from build123d import *

# Parameters (mm, degrees)
F1_DEPTH       = 10
F3_D           = 5
F3_CBORE_D     = 9
F3_CBORE_DEPTH = 1.5
F4_T1_DEPTH    = 10
F4_T3_DEPTH    = 10
F4_T5_DEPTH    = 10
F4_T7_DEPTH    = 35
F4_T9_DEPTH    = 35
F4_T11_DEPTH   = 35
F4_T13_DEPTH   = 34.4948974279
F5_R           = 2


# Not quite as in the source:
# - a fillet or chamfer that OpenCascade refuses, or shapes differently, is made with other operations: its cross-section is extruded or revolved along the edge and cut away or added


with BuildPart() as f1:
    # F0 (on Top) → F1 (new body)
    with BuildSketch(Plane.XY):
        Polygon((-60, 0), (0, 0), (0, 7), (-54, 7), (-54, 22), (-20, 22), (-20, 11), (-16, 11), (-16, 28), (-60, 28), align=None)
    extrude(amount=F1_DEPTH)

    # F3 (through all)
    with Locations(Plane(origin=(0, 7, 0), x_dir=(-1, 0, 0), z_dir=(0, 1, 0))):
        with Locations((8, 5)):
            CounterBoreHole(F3_D / 2, F3_CBORE_D / 2, F3_CBORE_DEPTH)

    # F4: fillet of radius 5 on 7 edges, made by hand

    # F4_s2 → F4_t1 (join)
    with BuildSketch(Plane.XY):
        with BuildLine():
            ThreePointArc((-49, 7), (-52.5355339059, 8.4644660941), (-54, 12))
            Line((-54, 12), (-54, 7))
            Line((-54, 7), (-49, 7))
        make_face()
    extrude(amount=F4_T1_DEPTH)

    # F4_s4 → F4_t3 (join)
    with BuildSketch(Plane.XY):
        with BuildLine():
            ThreePointArc((-54, 17), (-52.5355339059, 20.5355339059), (-49, 22))
            Line((-49, 22), (-54, 22))
            Line((-54, 22), (-54, 17))
        make_face()
    extrude(amount=F4_T3_DEPTH)

    # F4_s6 → F4_t5 (join)
    with BuildSketch(Plane.XY):
        with BuildLine():
            ThreePointArc((-25, 22), (-21.4644660941, 20.5355339059), (-20, 17))
            Line((-20, 17), (-20, 22))
            Line((-20, 22), (-25, 22))
        make_face()
    extrude(amount=F4_T5_DEPTH)

    # F4_s8 → F4_t7 (cut)
    with BuildSketch(Plane.XY.offset(-12.5)):
        with BuildLine():
            ThreePointArc((-55, 0), (-58.5355339059, 1.4644660941), (-60, 5))
            Line((-60, 5), (-60, 0))
            Line((-60, 0), (-55, 0))
        make_face()
    extrude(amount=F4_T7_DEPTH, mode=Mode.SUBTRACT)

    # F4_s10 → F4_t9 (cut)
    with BuildSketch(Plane.XY.offset(-12.5)):
        with BuildLine():
            ThreePointArc((-60, 23), (-58.5355339059, 26.5355339059), (-55, 28))
            Line((-55, 28), (-60, 28))
            Line((-60, 28), (-60, 23))
        make_face()
    extrude(amount=F4_T9_DEPTH, mode=Mode.SUBTRACT)

    # F4_s12 → F4_t11 (cut)
    with BuildSketch(Plane.XY.offset(-12.5)):
        with BuildLine():
            ThreePointArc((-21, 28), (-17.4644660941, 26.5355339059), (-16, 23))
            Line((-16, 23), (-16, 28))
            Line((-16, 28), (-21, 28))
        make_face()
    extrude(amount=F4_T11_DEPTH, mode=Mode.SUBTRACT)

    # F4_s14 → F4_t13 (cut)
    with BuildSketch(Plane.XY.offset(-12.2474487139)):
        with BuildLine():
            ThreePointArc((-16, 15.8989794856), (-17.1270166538, 12.7367018254), (-20, 11))
            Line((-20, 11), (-16, 11))
            Line((-16, 11), (-16, 15.8989794856))
        make_face()
    extrude(amount=F4_T13_DEPTH, mode=Mode.SUBTRACT)

    # F5
    f5_edges = [f1.edges().sort_by_distance(p)[0] for p in [
        (-38, 28, 0),
        (-55, 28, 5),
        (-38, 28, 10),
        (-21, 28, 5),
        (-16, 19.44949, 0),
        (-16, 19.44949, 10),
        (-60, 14, 0),
        (-60, 14, 10),
        (-27.5, 0, 0),
        (-27.5, 0, 10),
        (-58.535534, 1.464466, 0),
        (-58.535534, 26.535534, 0),
        (-17.464466, 26.535534, 0),
        (-17.127017, 12.736702, 0),
        (-58.535534, 1.464466, 10),
        (-58.535534, 26.535534, 10),
        (-17.464466, 26.535534, 10),
        (-17.127017, 12.736702, 10),
    ]]
    fillet(f5_edges, radius=F5_R)


solid = f1.part
Could you check a few things on this model? Use its own coordinates, in mm. A direction names the side the tool comes from. Give positions to 0.01 mm unless a question says otherwise; leave off trailing zeros. Order: outer loops, then holes, each group sorted by start corner. A loop starts at its lowest first (then second) coordinate and runs counter-clockwise, first axis right, second up. Notation, with made-up numbers: (56.5, 60.25) - (88.5, 60.25) arc R16 cw to (88.5, 85.25) - close; hole circle Ø2 at (26.25, 35.5). An arc over 180 degrees is marked (long way). One line per question, with ' | ' between items. Start each with the question number.
Item 1: I want a section at A-A on z = 5. Write out the boundary of the cut face in (x, y), then the cut area to 3 significant figures.
Item 2: I want a section at B-B on x = -47. Write out the boundary of the cut face in (y, z), then the cut area to 3 significant figures.
Item 3: I want a section at D-D on x = -8. Write out the boundary of the cut face in (y, z), then the cut area to 3 significant figures.
Item 4: For faces 4 (the cylindrical face through (-16.6, 19.5, 0.57)), 5 (the cylindrical face through (-12.16, 6.26, 3.28)), 6 (the flat face through (-16, 19, 5)), 7 (the cylindrical face through (-17.1, 12.77, 4.96)), 8 (the flat face through (-20, 14, 5)), which set-ups out of +Z, -Z, +X, -X, +Y, -Y let a thin tool reach every point of the face, with its end or its side?
Item 5: I'm going to push flat-ended pins straight in: pin 1 Ø4 at (y, z) = (23.5, 6.5) entering from +X; pin 2 Ø4 at (x, z) = (-51, 5) entering from -Y; pin 3 Ø2.5 at (x, z) = (-10, 6.5) entering from +Y; pin 4 Ø5 at (x, z) = (-14.5, 6.5) entering from +Y. Where does each tip first touch, or does it pass through?
Item 6: I want a section at C-C on y = 20.75. Write out the boundary of the cut face in (x, z).
Item 7: I need wall thicknesses on probe 1 along Z at (x, y) = (-8, 2.85); probe 2 along Y at (x, z) = (-39.5, 2.5); probe 3 along Z at (x, y) = (-8, 6.2). Which ranges of each line are inside material? Lowest first, please. Write a range as [from, to].
Item 8: Thinking about a two-plate mould opening in Y: for faces 1 (the cylindrical face through (-9.84, 2.71, 6.69)), 2 (the cylindrical face through (-53, 20, 5)), 3 (the flat face through (-10, 5.5, 3)), which applies, pulls with the +Y half, pulls with the -Y half, needs draft (parallel to the pull), parting line crosses it, or undercut?
Verdict:
1) outline: (-60, 5) arc R5 ccw to (-55, 0) - (-10.5, 0) - (-10.5, 5.5) - (-12.5, 5.5) - (-12.5, 7) - (-49, 7) arc R5 cw to (-54, 12) - (-54, 17) arc R5 cw to (-49, 22) - (-25, 22) arc R5 cw to (-20, 17) - (-20, 11) arc R5 ccw to (-16, 15.9) - (-16, 23) arc R5 ccw to (-21, 28) - (-55, 28) arc R5 ccw to (-60, 23) - close; (-5.5, 0) - (0, 0) - (0, 7) - (-3.5, 7) - (-3.5, 5.5) - (-5.5, 5.5) - close | area: 772 mm^2
2) outline: (0, 2) arc R2 ccw to (2, 0) - (7, 0) - (7, 10) - (2, 10) arc R2 ccw to (0, 8) - close; (22, 0) - (26, 0) arc R2 ccw to (28, 2) - (28, 8) arc R2 ccw to (26, 10) - (22, 10) - close | area: 127 mm^2
3) outline: (0, 2) arc R2 ccw to (2, 0) - (7, 0) - (7, 0.5) - (5.5, 0.5) - (5.5, 2.5) - (0, 2.5) - close; (0, 7.5) - (5.5, 7.5) - (5.5, 9.5) - (7, 9.5) - (7, 10) - (2, 10) arc R2 ccw to (0, 8) - close | area: 27.3 mm^2
4) face 4: -Z, +X, +Y | face 5: +Y | face 6: +Z, -Z, +X, +Y | face 7: +Z, -Z, +X | face 8: +Z, -Z
5) pin 1: x = -16 | pin 2: y = 0 | pin 3: y = 5.5 | pin 4: y = 26
6) outline: (-60, 2) arc R2 ccw to (-58, 0) - (-52.31, 0) - (-52.31, 10) - (-58, 10) arc R2 ccw to (-60, 8) - close; (-21.69, 0) - (-18, 0) arc R2 ccw to (-16, 2) - (-16, 8) arc R2 ccw to (-18, 10) - (-21.69, 10) - close
7) probe 1: [0, 2.5], [7.5, 10] | probe 2: [0, 7], [22, 28] | probe 3: [0, 0.5], [9.5, 10]
8) face 1: needs draft | face 2: undercut | face 3: pulls with the +Y half
